```python
from build123d import *

# Parameters (mm, degrees)
WIDE_FLANGE_WITH_ORIGINAL_FLOOR_BOLT_2_R       = 2.75
WIDE_FLANGE_WITH_ORIGINAL_FLOOR_BOLT_CEN_DEPTH = 1


with BuildPart() as part:
    # Wide flange with original floor bolt 2 → Wide flange with original floor bolt cen (new body)
    with BuildSketch(Plane.XY):
        Polygon((-97.5, -14.5), (97.5, -14.5), (97.5, -5), (94, -1.5), (94, 0), (-97.5, 0), align=None)
        with Locations((-90, -9)):
            Circle(WIDE_FLANGE_WITH_ORIGINAL_FLOOR_BOLT_2_R, mode=Mode.SUBTRACT)
        with Locations((-31, -9)):
            Circle(WIDE_FLANGE_WITH_ORIGINAL_FLOOR_BOLT_2_R, mode=Mode.SUBTRACT)
        with Locations((31, -9)):
            Circle(WIDE_FLANGE_WITH_ORIGINAL_FLOOR_BOLT_2_R, mode=Mode.SUBTRACT)
        with Locations((90, -9)):
            Circle(WIDE_FLANGE_WITH_ORIGINAL_FLOOR_BOLT_2_R, mode=Mode.SUBTRACT)
    extrude(amount=WIDE_FLANGE_WITH_ORIGINAL_FLOOR_BOLT_CEN_DEPTH)


solid = part.part
```
Could you check a few things on this model? Use its own coordinates, in mm. Coordinates: 2 decimals unless noted, no trailing zeros. Order: outer loops, then holes, each group sorted by start corner. A loop starts at its lowest first (then second) coordinate and runs counter-clockwise, first axis right, second up. Notation, with made-up numbers: M 79,-13 L 138,-13 A27 ccw 138,5 Z; hole C 42,-4 d4. An arc over 180 degrees is marked long. Use a Markdown table: item, result. Add a question column.
Q1. If I drill on L1, parallel to X at y = -8, z = 0.4; L2, parallel to Y at x = 31, z = 0.3; L3, parallel to X at y = -9.5, z = 0.35, over which ranges is the centre line in solid material (lowest first)?
Q2. I'm going to push a flat-ended pin straight in: pin 1 (0.5 mm diameter, centred on y = -0.5, z = 0.5, fed in from +X). Where does the tip first touch, or does it pass through?
Q3. We'd pull the mould along X, two halves only. Please class faces 1 (the flat face through (95.8, -3.3, 0.5)), 2 (the flat face through (-1, -7, 1)), 3 (the cylindrical face through (-92.747, -8.879, 0.493)): pulls with the +X half, pulls with the -X half, needs draft (parallel to the pull), parting line crosses it, or undercut.
Q4. I want a section at C-C on z = 0.2. List the corners of the cut face in (x, y) for me, then the cut area to 3 significant figures.
Q5. I want a section at B-B on x = 31. List the corners of the cut face in (y, z) for me, then the cut area to 3 significant figures.
Q6. I want a section at A-A on y = -9. List the corners of the cut face in (x, z) for me, then the cut area to 3 significant figures.
Checked values:
| question | item | result |
|---|---|---|
| 1 | L1 | -97.5 to -92.56, -87.44 to -33.56, -28.44 to 28.44, 33.56 to 87.44, 92.56 to 97.5 |
| 1 | L2 | -14.5 to -11.75, -6.25 to 0 |
| 1 | L3 | -97.5 to -92.7, -87.3 to -33.7, -28.3 to 28.3, 33.7 to 87.3, 92.7 to 97.5 |
| 2 | pin 1 | x = 94 |
| 3 | face 1 | pulls with the +X half |
| 3 | face 2 | needs draft |
| 3 | face 3 | undercut |
| 4 | outline | M -97.5,-14.5 L 97.5,-14.5 L 97.5,-5 L 94,-1.5 L 94,0 L -97.5,0 Z; hole C -90,-9 d5.5; hole C -31,-9 d5.5; hole C 31,-9 d5.5; hole C 90,-9 d5.5 |
| 4 | area | 2,720 mm² |
| 5 | outline | M -14.5,0 L -11.75,0 L -11.75,1 L -14.5,1 Z; M -6.25,0 L 0,0 L 0,1 L -6.25,1 Z |
| 5 | area | 9.00 mm² |
| 6 | outline | M -97.5,0 L -92.75,0 L -92.75,1 L -97.5,1 Z; M -87.25,0 L -33.75,0 L -33.75,1 L -87.25,1 Z; M -28.25,0 L 28.25,0 L 28.25,1 L -28.25,1 Z; M 33.75,0 L 87.25,0 L 87.25,1 L 33.75,1 Z; M 92.75,0 L 97.5,0 L 97.5,1 L 92.75,1 Z |
| 6 | area | 173 mm² |
